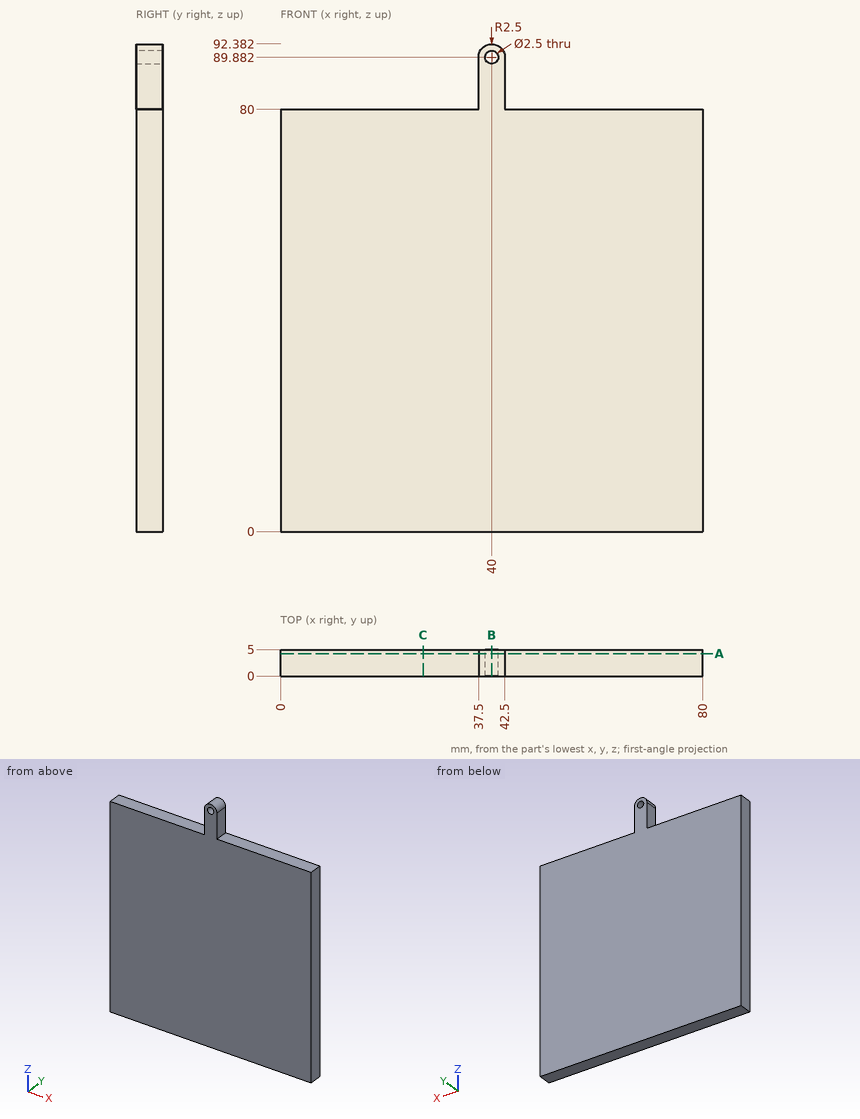
Can you work these out from the drawing? Everything is in mm from the part's minimum corner. Coordinates: 2 decimals unless noted, no trailing zeros. Loops run counter-clockwise (first coordinate to the right, second up) from the corner with the lowest first, then second, coordinate; pieces in that order, holes last.
1) I need wall thicknesses on probe 1 along Z at (x, y) = (66, 0.8); probe 2 along X at (y, z) = (3.15, 84); probe 3 along Z at (x, y) = (38, 0.9). Which ranges of each line are inside material? Lowest first, please.
2) Imagine slicing it at B-B on x = 40. List the corners of the cut face in (y, z) for me.
3) Imagine slicing it at C-C on x = 27. List the corners of the cut face in (y, z) for me, plus the area to 3 significant figures.
4) Imagine slicing it at A-A on y = 4.25. List the corners of the cut face in (x, z) for me.
5) For pin 1 (1.5 mm diameter, centred on y = 1.5, z = 82.5, fed in from -X); pin 2 (2.5 mm diameter, centred on x = 66.5, y = 2, fed in from +Z); pin 3 (1.5 mm diameter, centred on x = 40, z = 89.88, fed in from +Y), each with a flat end and sliding along its axis, tell me the tip position at first contact or that it passes through.
Completed:
1. probe 1: z = 0 to 80
1. probe 2: x = 37.5 to 42.5
1. probe 3: z = 0 to 91.38
2. outline: (0, 0) - (5, 0) - (5, 88.63) - (0, 88.63) - close; (0, 91.13) - (5, 91.13) - (5, 92.38) - (0, 92.38) - close
3. outline: (0, 0) - (5, 0) - (5, 80) - (0, 80) - close
3. area: 400 mm2
4. outline: (0, 0) - (80, 0) - (80, 80) - (42.5, 80) - (42.5, 89.88) arc R2.5 ccw to (37.5, 89.88) - (37.5, 80) - (0, 80) - close; hole circle Ø2.5 at (40, 89.88)
5. pin 1: stops at x = 37.5
5. pin 2: stops at z = 80
5. pin 3: passes through
